Build history of the part. All positions in model axes, mm. Face numbers are marked on the shaded views. A direction names the side the tool comes from. Give positions to 0.01 mm unless a question says otherwise; leave off trailing zeros. Loops run counter-clockwise (first coordinate to the right, second up) from the corner with the lowest first, then second, coordinate; pieces in that order, holes last. Notation, with made-up numbers: M -39,12.5 L -25,12.5 A18 ccw -25,28.5 Z; hole C -23.75,-18 d1. An arc over 180 degrees is marked long. Answer as a JSON object with one key per item and string values. Group by question number.
1. Slice it at D-D (x = -1). List the corners of the cut face in (y, z).
2. Slice it at A-A (x = 1). List the corners of the cut face in (y, z).
3. Slice it at C-C (y = 1.5). List the corners of the cut face in (x, z).
4. Mould opens along Z. For the marked faces 3, 4 and 5 say: released by +Z, released by -Z, zero draft, split by the parting line, or undercut.
5. Slice it at B-B (z = 2.5). List the corners of the cut face in (x, y), then the cut area to 3 significant figures.
6. Drill centre lines: line 1 along X through (y, z) = (7.75, -7.5); line 2 along Z through (x, y) = (0.5, 8.5); line 3 along Z through (x, y) = (-4.75, 3.75). Where is each one in solid material? Low to high. Write a range as [from, to].
7. 3-axis set-ups, long thin cutter, end or side, ignore diameter. For the marked faces 1 and 2: which of +Z, -Z, +X, -X, +Y, -Y reach the whole face in a straight line?
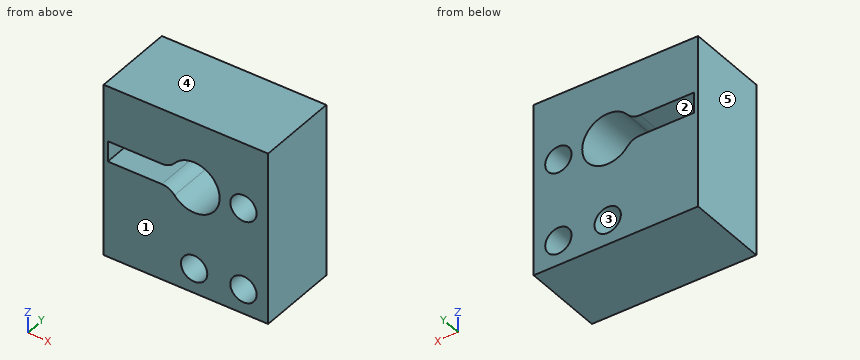
from build123d import *

# Parameters (mm, degrees)
SKETCH_1_W          = 20
SKETCH_1_H          = 21
EXTRUDE_1_DEPTH     = 10
CUT_EXTRUDE_1_DEPTH = 18.613914954
FILLET_2_R          = 2
SKETCH_3_R          = 1.6
CUT_EXTRUDE_2_DEPTH = 18.613914954
SKETCH_4_W          = 0.5
SKETCH_4_H          = 2.5
EXTRUDE_2_DEPTH     = 10


with BuildPart() as part:
    # 草图1 → 凸台-拉伸1 (new body)
    with BuildSketch(Plane(origin=(0, 0, 0), x_dir=(1, 0, 0), z_dir=(0, 1, 0))):
        Rectangle(SKETCH_1_W, SKETCH_1_H)
    extrude(amount=EXTRUDE_1_DEPTH)

    # 草图2 → 切除-拉伸1 (cut, through all)
    with BuildSketch(Plane(origin=(0, 10, 0), x_dir=(1, 0, 0), z_dir=(0, 1, 0))):
        with BuildLine():
            Line((-1.836811591, -1.25), (-10, -1.25))
            Line((-10, -1.25), (-10, -3.75))
            Line((-10, -3.75), (-1.836811591, -3.75))
            ThreePointArc((-1.836811591, -3.75), (4.1, -2.5), (-1.836811591, -1.25))
        make_face()
    extrude(amount=-CUT_EXTRUDE_1_DEPTH, mode=Mode.SUBTRACT)

    # 圆角2
    fillet_2_edges = [part.edges().sort_by_distance(p)[0] for p in [
        (-1.836811591, 5, 1.25),
        (-1.836811591, 5, 3.75),
    ]]
    fillet(fillet_2_edges, radius=FILLET_2_R)

    # 草图3 → 切除-拉伸2 (cut, through all)
    with BuildSketch(Plane(origin=(0, 10, 0), x_dir=(1, 0, 0), z_dir=(0, 1, 0))):
        with Locations(Location((1, 7.5, 0), (0, 0, 270))):
            Circle(SKETCH_3_R)
        with Locations(Location((7, 7.5, 0), (0, 0, 270))):
            Circle(SKETCH_3_R)
        with Locations(Location((7, -2.5, 0), (0, 0, 270))):
            Circle(SKETCH_3_R)
    extrude(amount=-CUT_EXTRUDE_2_DEPTH, mode=Mode.SUBTRACT)

    # 草图4 → 凸台-拉伸2 (add)
    with BuildSketch(Plane(origin=(0, 10, 0), x_dir=(1, 0, 0), z_dir=(0, 1, 0))):
        with Locations((-9.75, -2.5)):
            Rectangle(SKETCH_4_W, SKETCH_4_H)
    extrude(amount=-EXTRUDE_2_DEPTH)


solid = part.part
Established:
{
 "1": {"outline": "M 0,-10.5 L 10,-10.5 L 10,0.13 L 0,0.13 Z; M 0,4.87 L 10,4.87 L 10,10.5 L 0,10.5 Z"},
 "2": {"outline": "M 0,-10.5 L 10,-10.5 L 10,-9.1 L 0,-9.1 Z; M 0,-5.9 L 10,-5.9 L 10,-0.6 L 0,-0.6 Z; M 0,5.6 L 10,5.6 L 10,10.5 L 0,10.5 Z"},
 "3": {"outline": "M -10,-10.5 L 10,-10.5 L 10,10.5 L -10,10.5 Z; hole M -9.5,1.25 L -2.93,1.25 A2 cw -1.39,0.52 A3.1 ccw long -1.39,4.48 A2 cw -2.93,3.75 L -9.5,3.75 Z; hole C 1,-7.5 d3.2; hole C 7,-7.5 d3.2; hole C 7,2.5 d3.2"},
 "4": {"face 3": "undercut", "face 4": "released by +Z", "face 5": "zero draft"},
 "5": {"outline": "M -10,0 L -9.5,0 L -9.5,10 L -10,10 Z; M 4.1,0 L 5.4,0 L 5.4,10 L 4.1,10 Z; M 8.6,0 L 10,0 L 10,10 L 8.6,10 Z", "area": "32.0 mm^2"},
 "6": {"line 1": "x = [-10, -0.6], [2.6, 5.4], [8.6, 10]", "line 2": "z = [-10.5, -9.02], [-5.98, -0.56], [5.56, 10.5]", "line 3": "z = [-10.5, 1.25], [3.75, 10.5]"},
 "7": {"face 1": "+Z, -Z, +X, -X, -Y", "face 2": "+Y, -Y"}
}
